Check sheet for the modelled part. Datum: model origin and axes. Units: mm. A direction names the side the tool comes from. Round coordinates to 2 decimals unless told otherwise and drop trailing zeros. Loops run counter-clockwise (first coordinate to the right, second up) from the corner with the lowest first, then second, coordinate; pieces in that order, holes last. Notation, with made-up numbers: (67, 22.5) -> (72, 22.5) arc R15 cw to (72, 32.5) -> close; hole circle Ø2 at (-9.75, -25.5). An arc over 180 degrees is marked (long way). Return JSON: item names as keys, results as strings.
from build123d import *

# Parameters (mm, degrees)
F1_DEPTH = 40
F3_D     = 6.5
F3_DEPTH = 30
F4_R     = 2


with BuildPart() as f1:
    # F0 (on Front) → F1 (new body)
    with BuildSketch(Plane.XZ):
        Polygon((0, 11.5), (0, 0), (60, 0), (60, 5), (30, 5), (30, 11.5), align=None)
    extrude(amount=F1_DEPTH)

    # F3
    with Locations(Plane.XY.offset(5)):
        with Locations((45, -20)):
            Hole(F3_D / 2, depth=F3_DEPTH)

    # F4
    f4_edges = [f1.edges().sort_by_distance(p)[0] for p in [
        (0, -20, 11.5),
        (15, -40, 11.5),
        (30, -20, 11.5),
        (15, 0, 11.5),
        (0, 0, 5.75),
        (0, -40, 5.75),
        (30, -40, 8.25),
        (30, 0, 8.25),
        (45, -40, 5),
        (60, -20, 5),
        (45, 0, 5),
        (60, -40, 2.5),
        (60, 0, 2.5),
        (30, -40, 0),
        (0, -20, 0),
        (30, 0, 0),
        (60, -20, 0),
    ]]
    fillet(f4_edges, radius=F4_R)


solid = f1.part
Q1. Tool access check on faces 1 (the cylindrical face through (0.57, -20.25, 0.6)), 2 (the cylindrical face through (0.57, -0.6, 5.7)), 3 (the cylindrical face through (42.79, -0.57, 4.4)), 4 (the cylindrical face through (29.4, -39.43, 7.02)), 5 (the flat face through (30, -20, 7)). Record the directions out of +Z, -Z, +X, -X, +Y, -Y that give a thin tool (end or side, any length) a straight path to the whole face; none if there is none.
Results list:
{"face 1": "-Z, -X, +Y, -Y", "face 2": "+Z, -Z, -X, +Y", "face 3": "+Z, +X, +Y", "face 4": "+Z, +X, -Y", "face 5": "+Z, +X, +Y, -Y"}
Q2. Section check A-A (x = 45). Record the boundary of the cut face in (y, z), then the cut area to 3 significant figures.
Results list:
{"outline": "(-40, 2) arc R2 ccw to (-38, 0) -> (-23.25, 0) -> (-23.25, 5) -> (-38, 5) arc R2 ccw to (-40, 3) -> close; (-16.75, 0) -> (-2, 0) arc R2 ccw to (0, 2) -> (0, 3) arc R2 ccw to (-2, 5) -> (-16.75, 5) -> close", "area": "164 mm^2"}
Q3. Section check C-C (y = -10). Record the boundary of the cut face in (x, z).
Results list:
{"outline": "(0, 2) arc R2 ccw to (2, 0) -> (58, 0) arc R2 ccw to (60, 2) -> (60, 3) arc R2 ccw to (58, 5) -> (30, 5) -> (30, 9.5) arc R2 ccw to (28, 11.5) -> (2, 11.5) arc R2 ccw to (0, 9.5) -> close"}
Q4. Section check B-B (x = 34). Record the boundary of the cut face in (y, z).
Results list:
{"outline": "(-40, 2) arc R2 ccw to (-38, 0) -> (-2, 0) arc R2 ccw to (0, 2) -> (0, 3) arc R2 ccw to (-2, 5) -> (-38, 5) arc R2 ccw to (-40, 3) -> close"}
Q5. Go/stop test with flat-tipped pins: pin 1 (4 mm diameter, centred on x = 45, y = -20, fed in from -Z); pin 2 (1 mm diameter, centred on y = -26, z = 10, fed in from -X); pin 3 (3.5 mm diameter, centred on y = -14.5, z = 6.5, fed in from +X); pin 4 (12 mm diameter, centred on x = 49, y = -29, fed in from +Z). Record where each tip stops, or that it passes through.
Results list:
{"pin 1": "through", "pin 2": "x = 0", "pin 3": "x = 58.97", "pin 4": "z = 5"}
Q6. Material ranges on line 1 (Y direction, x = 45, z = 2.4); line 2 (Z direction, x = 54.5, y = -5); line 3 (X direction, y = -17, z = 3.75), recorded low to high.
Results list:
{"line 1": "-40 to -23.25, -16.75 to 0", "line 2": "0 to 5", "line 3": "0 to 43.75, 46.25 to 59.85"}
